```python
from build123d import *

# Parameters (mm, degrees)
SKETCH_1_R      = 3.333333333
EXTRUDE_1_DEPTH = 2
SCALE_1_SCALE   = 1.5
CHAMFER_1_SIZE  = 0.2
FILLET_1_R      = 5
FILLET_2_R      = 1


with BuildPart() as part:
    # 草图1 → 凸台-拉伸1 (new body)
    with BuildSketch(Plane(origin=(0, 0, 0), x_dir=(1, 0, 0), z_dir=(0, 1, 0))):
        with BuildLine():
            Line((-4, -4.472135955), (-4, -113.07179677))
            ThreePointArc((-4, -113.07179677), (0, -128), (4, -113.07179677))
            Line((4, -113.07179677), (4, -4.472135955))
            ThreePointArc((4, -4.472135955), (0, 6), (-4, -4.472135955))
        make_face()
        with Locations(Location((0, 0, 0), (0, 0, 270))):
            Circle(SKETCH_1_R, mode=Mode.SUBTRACT)
        with Locations(Location((0, -120, 0), (0, 0, 270))):
            Circle(SKETCH_1_R, mode=Mode.SUBTRACT)
    extrude(amount=EXTRUDE_1_DEPTH)


with BuildPart() as part_1:
    # 缩放比例1: scaled about (0, 1, 63.97284267)
    add(part.part.scale(SCALE_1_SCALE).moved(Location((0, -0.5, -31.986421335))))

    # 倒角1
    chamfer_1_edges = [part_1.edges().sort_by_distance(p)[0] for p in [
        (0, 2.5, -36.986421335),
        (0, 2.5, 143.013578665),
    ]]
    chamfer(chamfer_1_edges, length=CHAMFER_1_SIZE)

    # 圆角1
    fillet_1_edges = [part_1.edges().sort_by_distance(p)[0] for p in [
        (6, 1, -25.278217403),
        (6, 1, 137.62127382),
        (-6, 1, 137.62127382),
        (-6, 1, -25.278217403),
    ]]
    fillet(fillet_1_edges, radius=FILLET_1_R)

    # 圆角2
    fillet_2_edges = [part_1.edges().sort_by_distance(p)[0] for p in [
        (6, 2.5, 55.862964986),
        (0, 2.5, 160.013578665),
        (-6, 2.5, 55.862964986),
        (0, 2.5, -40.986421335),
        (6.462573935, 2.5, 137.152517394),
        (-6.462573935, 2.5, 137.152517394),
        (-6.275444087, 2.5, -24.962801474),
        (6.275444087, 2.5, -24.962801474),
    ]]
    fillet(fillet_2_edges, radius=FILLET_2_R)


solid = part_1.part
```
Input: part model. Units: mm. Frame: model coordinates. Give positions to 0.01 mm unless a question says otherwise; leave off trailing zeros. Order: outer loops, then holes, each group sorted by start corner. A loop starts at its lowest first (then second) coordinate and runs counter-clockwise, first axis right, second up. Notation, with made-up numbers: (64.5, -14) - (75.5, -14) arc R22 ccw to (75.5, 24) - close; hole circle Ø4 at (-26, 59.5). An arc over 180 degrees is marked (long way). One line per item, written item: value.
1. Cut plane C-C, the plane z = 62.5. Output: boundary loops of the cut face in (x, y).
Determined:
outline: (-6, -0.5) - (6, -0.5) - (6, 1.5) arc R1 ccw to (5, 2.5) - (-5, 2.5) arc R1 ccw to (-6, 1.5) - close
2. Draft query along Z for faces 1 (the face through (-1.92, 0.88, 152.63)), 2 (the face through (0, 2.5, 58)). Return one class per face: released by +Z, released by -Z, zero draft, split by the parting line, or undercut.
Determined:
face 1: undercut
face 2: zero draft
3. Line query: probe 1 along Z at (x, y) = (-1.25, 2.15); probe 2 along Z at (x, y) = (2, 0.55); probe 3 along X at (y, z) = (0, 62). Output: solid intervals per line, ascending.
Determined:
probe 1: -40.66 to -36.83, -27.15 to 143.17, 152.85 to 159.71
probe 2: -40.76 to -36.57, -27.4 to 143.43, 152.6 to 159.85
probe 3: -6 to 6
4. Cut plane A-A, the plane x = 0. Output: boundary loops of the cut face in (y, z).
Determined:
outline: (-0.5, -40.99) - (1.5, -40.99) arc R1 ccw to (2.5, -39.99) - (2.5, -37.19) - (2.3, -36.99) - (-0.5, -36.99) - close; (-0.5, -26.99) - (2.3, -26.99) - (2.5, -26.79) - (2.5, 142.81) - (2.3, 143.01) - (-0.5, 143.01) - close; (-0.5, 153.01) - (2.3, 153.01) - (2.5, 153.21) - (2.5, 159.01) arc R1 ccw to (1.5, 160.01) - (-0.5, 160.01) - close
5. Pin query (flat end, axial travel): pin 1 Ø1 at (y, z) = (0.5, 94.5) entering from -X. Return the tip coordinate at first contact, or that it passes through.
Determined:
pin 1: x = -6
6. Cut plane B-B, the plane y = 0.05. Output: boundary loops of the cut face in (x, z).
Determined:
outline: (-7.76, 138.86) arc R5 cw to (-6, 135.05) - (-6, -23.33) arc R5 cw to (-7.07, -26.42) arc R9 ccw (long way) to (7.07, -26.42) arc R5 cw to (6, -23.33) - (6, 135.05) arc R5 cw to (7.76, 138.86) arc R12 ccw (long way) to start; hole circle Ø10 at (0, -31.99); hole circle Ø10 at (0, 148.01)
